Here's how the part is built. I have some questions about the finished solid (model axes, mm). Face numbers are marked on the shaded views. A direction names the side the tool comes from. Give positions to 0.01 mm unless a question says otherwise; leave off trailing zeros. Write each loop counter-clockwise with the first axis right and the second up, starting at its lowest first coordinate (ties: lowest second). Pieces come first, ordered by that corner, then holes. Notation, with made-up numbers: (1, 27) -> (48, 27) arc R22 ccw to (48, 60) -> close; hole circle Ø1 at (35.5, 69.25). An arc over 180 degrees is marked (long way). Put each result on its own line as item: value. Start each with the question number.
from build123d import *

# Parameters (mm, degrees)
BOSS_EXTRUDE1_DEPTH = 15
SKETCH2_R           = 20
CUT_EXTRUDE1_DEPTH  = 45
CUT_EXTRUDE2_DEPTH  = 10


with BuildPart() as part:
    # Sketch1 → Boss-Extrude1 (new, symmetric)
    with BuildSketch(Plane.XY):
        with BuildLine():
            Line((-53.25352101, 13.75), (-21.785531322, 135.625))
            ThreePointArc((-21.785531322, 135.625), (0, 152.5), (21.785531322, 135.625))
            Line((21.785531322, 135.625), (53.25352101, 13.75))
            ThreePointArc((53.25352101, 13.75), (0, -55), (-53.25352101, 13.75))
        make_face()
    extrude(amount=BOSS_EXTRUDE1_DEPTH, both=True)

    # Sketch2 → Cut-Extrude1 (cut)
    with BuildSketch(Plane.XY.offset(15)):
        with Locations((0, 130)):
            Circle(SKETCH2_R)
    extrude(amount=-CUT_EXTRUDE1_DEPTH, mode=Mode.SUBTRACT)

    # Sketch4 → Cut-Extrude2 (cut, symmetric)
    with BuildSketch(Plane.XY):
        with BuildLine():
            Line((-21.785531322, 135.625), (-35.020174222, 84.367448459))
            ThreePointArc((-35.020174222, 84.367448459), (0, 53.836754328), (35.020174222, 84.367448459))
            Line((35.020174222, 84.367448459), (21.785531322, 135.625))
            ThreePointArc((21.785531322, 135.625), (0, 152.5), (-21.785531322, 135.625))
        make_face()
    extrude(amount=CUT_EXTRUDE2_DEPTH, both=True, mode=Mode.SUBTRACT)


solid = part.part
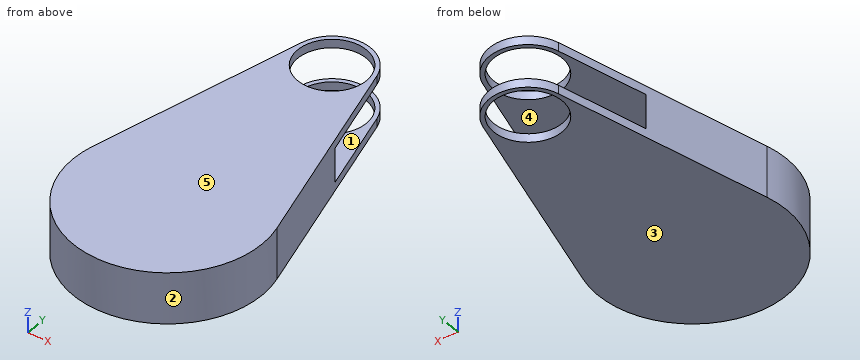
1) Which directions (+Z, -Z, +X, -X, +Y, -Y) give clear straight access to the entire face, cutting with the end or side of a thin tool? Please do the marked faces 4 and 5.
2) Thinking about a two-plate mould opening in X: for the marked faces 1, 2 and 3, which applies, released by +X, released by -X, zero draft, split by the parting line, or undercut?
3) I want a section at A-A, the plane x = 0. Write out the boundary of the cut face in (y, z).
4) I want a section at B-B, the plane y = 66.5. Write out the boundary of the cut face in (x, z).
5) I need wall thicknesses on probe 1 along Z at (x, y) = (-20, 85); probe 2 along X at (y, z) = (69, -3.5); probe 3 along X at (y, z) = (31.5, -4.5). Which ranges of each line are inside material? Lowest first, please.
6) I want a section at C-C, the plane y = 130. Write out the boundary of the cut face in (x, z).
7) I want a section at D-D, the plane z = 12.5. Write out the boundary of the cut face in (x, y) (3 decimals), and give its area (3 significant figures).
8) I'm going to push flat-ended pins straight in: pin 1 Ø6 at (y, z) = (24, 6.5) entering from -X; pin 2 Ø1 at (y, z) = (71, 11.5) entering from +X; pin 3 Ø6 at (x, z) = (-37.5, -10.5) entering from -Y. Where does each tip first touch, or does it pass through?
Established:
1. face 4: +Y
1. face 5: +Z, +X, -X, +Y, -Y
2. face 1: undercut
2. face 2: split by the parting line
2. face 3: zero draft
3. outline: (-55, -15) -> (110, -15) -> (110, -10) -> (53.84, -10) -> (53.84, 10) -> (110, 10) -> (110, 15) -> (-55, 15) -> close; (150, -15) -> (152.5, -15) -> (152.5, -10) -> (150, -10) -> close; (150, 10) -> (152.5, 10) -> (152.5, 15) -> (150, 15) -> close
4. outline: (-39.63, -15) -> (39.63, -15) -> (39.63, 15) -> (-39.63, 15) -> close; hole (-27.11, -10) -> (27.11, -10) -> (27.11, 10) -> (-27.11, 10) -> close
5. probe 1: z = -15 to -10, 10 to 15
5. probe 2: x = -38.99 to -29.02, 29.02 to 38.99
5. probe 3: x = -48.67 to 48.67
6. outline: (-23.24, -15) -> (-20, -15) -> (-20, -10) -> (-23.24, -10) -> close; (-23.24, 10) -> (-20, 10) -> (-20, 15) -> (-23.24, 15) -> close; (20, -15) -> (23.24, -15) -> (23.24, -10) -> (20, -10) -> close; (20, 10) -> (23.24, 10) -> (23.24, 15) -> (20, 15) -> close
7. outline: (-53.254, 13.75) arc R55 ccw (long way) to (53.254, 13.75) -> (21.786, 135.625) arc R22.5 ccw to (-21.786, 135.625) -> close; hole circle Ø40 at (0, 130)
7. area: 14,700 mm2
8. pin 1: stops at x = -51.38
8. pin 2: stops at x = 38.6
8. pin 3: stops at y = -42.83
